The listing builds one solid part. Answer for the finished solid, in the listing's coordinates (mm). A direction names the side the tool comes from. Give positions to 0.01 mm unless a question says otherwise; leave off trailing zeros. Answer as a JSON object with one key per item and string values. Group by question number.
```python
from build123d import *

# Parameters (mm, degrees)
BOSS_EXTRUDE1_DEPTH = 102.5
FILLET1_R           = 1
CUT_EXTRUDE1_DEPTH  = 103.5
FILLET2_R           = 0.5
FILLET3_R           = 0.25


with BuildPart() as part:
    # Sketch3 → Boss-Extrude1 (new body)
    with BuildSketch(Plane(origin=(0, 0, 0), x_dir=(1, 0, 0), z_dir=(0, 1, 0))):
        with BuildLine():
            Line((7, 18.5), (7, 19.5))
            ThreePointArc((7, 19.5), (6.646446609, 19.646446609), (6.5, 20))
            Line((6.5, 20), (0, 20))
            Line((0, 20), (0, 13.5))
            ThreePointArc((0, 13.5), (0.353553391, 13.353553391), (0.5, 13))
            Line((0.5, 13), (1.5, 13))
            Line((1.5, 13), (1.5, 16))
            Line((1.5, 16), (3, 16))
            Line((3, 16), (5.5, 13.5))
            Line((5.5, 13.5), (5.5, 10.5))
            Line((5.5, 10.5), (6, 10))
            Line((6, 10), (5.5, 9.5))
            Line((5.5, 9.5), (5.5, 6.5))
            Line((5.5, 6.5), (3, 4))
            Line((3, 4), (1.5, 4))
            Line((1.5, 4), (1.5, 7))
            Line((1.5, 7), (0.5, 7))
            ThreePointArc((0.5, 7), (0.353553391, 6.646446609), (0, 6.5))
            Line((0, 6.5), (0, 0))
            Line((0, 0), (6.5, 0))
            ThreePointArc((6.5, 0), (6.646446609, 0.353553391), (7, 0.5))
            Line((7, 0.5), (7, 1.5))
            Line((7, 1.5), (4, 1.5))
            Line((4, 1.5), (4, 3))
            Line((4, 3), (6.5, 5.5))
            Line((6.5, 5.5), (9.5, 5.5))
            Line((9.5, 5.5), (10, 6))
            Line((10, 6), (10.5, 5.5))
            Line((10.5, 5.5), (13.5, 5.5))
            Line((13.5, 5.5), (16, 3))
            Line((16, 3), (16, 1.5))
            Line((16, 1.5), (13, 1.5))
            Line((13, 1.5), (13, 0.5))
            ThreePointArc((13, 0.5), (13.353553391, 0.353553391), (13.5, 0))
            Line((13.5, 0), (20, 0))
            Line((20, 0), (20, 6.5))
            ThreePointArc((20, 6.5), (19.646446609, 6.646446609), (19.5, 7))
            Line((19.5, 7), (18.5, 7))
            Line((18.5, 7), (18.5, 4))
            Line((18.5, 4), (17, 4))
            Line((17, 4), (14.5, 6.5))
            Line((14.5, 6.5), (14.5, 9.5))
            Line((14.5, 9.5), (14, 10))
            Line((14, 10), (14.5, 10.5))
            Line((14.5, 10.5), (14.5, 13.5))
            Line((14.5, 13.5), (17, 16))
            Line((17, 16), (18.5, 16))
            Line((18.5, 16), (18.5, 13))
            Line((18.5, 13), (19.5, 13))
            ThreePointArc((19.5, 13), (19.646446609, 13.353553391), (20, 13.5))
            Line((20, 13.5), (20, 20))
            Line((20, 20), (13.5, 20))
            ThreePointArc((13.5, 20), (13.353553391, 19.646446609), (13, 19.5))
            Line((13, 19.5), (13, 18.5))
            Line((13, 18.5), (16, 18.5))
            Line((16, 18.5), (16, 17))
            Line((16, 17), (13.5, 14.5))
            Line((13.5, 14.5), (10.5, 14.5))
            Line((10.5, 14.5), (10, 14))
            Line((10, 14), (9.5, 14.5))
            Line((9.5, 14.5), (6.5, 14.5))
            Line((6.5, 14.5), (4, 17))
            Line((4, 17), (4, 18.5))
            Line((4, 18.5), (7, 18.5))
        make_face()
    extrude(amount=BOSS_EXTRUDE1_DEPTH)

    # Fillet1
    fillet1_edges = [part.edges().sort_by_distance(p)[0] for p in [
        (20, 51.25, 0),
        (0, 51.25, 0),
        (0, 51.25, -20),
        (20, 51.25, -20),
    ]]
    fillet(fillet1_edges, radius=FILLET1_R)

    # Sketch4 → Cut-Extrude1 (cut, through all)
    with BuildSketch(Plane(origin=(0, 102.5, 0), x_dir=(1, 0, 0), z_dir=(0, 1, 0))):
        with BuildLine():
            Line((10, 11), (11.195582496, 12.195582496))
            ThreePointArc((11.195582496, 12.195582496), (10, 12.5), (8.804417504, 12.195582496))
            Line((8.804417504, 12.195582496), (10, 11))
        make_face()
        with BuildLine():
            ThreePointArc((12.195582496, 11.195582496), (11.767766953, 11.767766953), (11.195582496, 12.195582496))
            Line((11.195582496, 12.195582496), (10, 11))
            Line((10, 11), (11, 10))
            Line((11, 10), (12.195582496, 11.195582496))
        make_face()
        with BuildLine():
            Line((9, 10), (10, 11))
            Line((10, 11), (8.804417504, 12.195582496))
            ThreePointArc((8.804417504, 12.195582496), (8.232233047, 11.767766953), (7.804417504, 11.195582496))
            Line((7.804417504, 11.195582496), (9, 10))
        make_face()
        Polygon((11, 10), (10, 11), (9, 10), (10, 9), align=None)
        with BuildLine():
            Line((7.804417504, 8.804417504), (9, 10))
            Line((9, 10), (7.804417504, 11.195582496))
            ThreePointArc((7.804417504, 11.195582496), (7.5, 10), (7.804417504, 8.804417504))
        make_face()
        with BuildLine():
            Line((10, 9), (9, 10))
            Line((9, 10), (7.804417504, 8.804417504))
            ThreePointArc((7.804417504, 8.804417504), (8.232233047, 8.232233047), (8.804417504, 7.804417504))
            Line((8.804417504, 7.804417504), (10, 9))
        make_face()
        with BuildLine():
            Line((11.195582496, 7.804417504), (10, 9))
            Line((10, 9), (8.804417504, 7.804417504))
            ThreePointArc((8.804417504, 7.804417504), (10, 7.5), (11.195582496, 7.804417504))
        make_face()
        with BuildLine():
            Line((12.195582496, 8.804417504), (11, 10))
            Line((11, 10), (10, 9))
            Line((10, 9), (11.195582496, 7.804417504))
            ThreePointArc((11.195582496, 7.804417504), (11.767766953, 8.232233047), (12.195582496, 8.804417504))
        make_face()
        with BuildLine():
            ThreePointArc((12.5, 10), (12.422700584, 10.616864556), (12.195582496, 11.195582496))
            Line((12.195582496, 11.195582496), (11, 10))
            Line((11, 10), (12.195582496, 8.804417504))
            ThreePointArc((12.195582496, 8.804417504), (12.422700584, 9.383135444), (12.5, 10))
        make_face()
        with BuildLine():
            ThreePointArc((8.804417504, 7.804417504), (8.232233047, 8.232233047), (7.804417504, 8.804417504))
            Line((7.804417504, 8.804417504), (7, 8))
            Line((7, 8), (8, 7))
            Line((8, 7), (8.804417504, 7.804417504))
        make_face()
        with BuildLine():
            Line((13, 8), (12.195582496, 8.804417504))
            ThreePointArc((12.195582496, 8.804417504), (11.767766953, 8.232233047), (11.195582496, 7.804417504))
            Line((11.195582496, 7.804417504), (12, 7))
            Line((12, 7), (13, 8))
        make_face()
        with BuildLine():
            Line((13, 12), (12, 13))
            Line((12, 13), (11.195582496, 12.195582496))
            ThreePointArc((11.195582496, 12.195582496), (11.767766953, 11.767766953), (12.195582496, 11.195582496))
            Line((12.195582496, 11.195582496), (13, 12))
        make_face()
        with BuildLine():
            ThreePointArc((7.804417504, 11.195582496), (8.232233047, 11.767766953), (8.804417504, 12.195582496))
            Line((8.804417504, 12.195582496), (8, 13))
            Line((8, 13), (7, 12))
            Line((7, 12), (7.804417504, 11.195582496))
        make_face()
    extrude(amount=-CUT_EXTRUDE1_DEPTH, mode=Mode.SUBTRACT)

    # Fillet2
    fillet2_edges = [part.edges().sort_by_distance(p)[0] for p in [
        (18.5, 51.25, -13),
        (18.5, 51.25, -16),
        (14.5, 51.25, -10.5),
        (14.5, 51.25, -9.5),
        (18.5, 51.25, -4),
        (18.5, 51.25, -7),
        (13, 51.25, -1.5),
        (16, 51.25, -1.5),
        (10.5, 51.25, -5.5),
        (9.5, 51.25, -5.5),
        (4, 51.25, -1.5),
        (7, 51.25, -1.5),
        (1.5, 51.25, -7),
        (1.5, 51.25, -4),
        (5.5, 51.25, -9.5),
        (5.5, 51.25, -10.5),
        (1.5, 51.25, -16),
        (1.5, 51.25, -13),
        (7, 51.25, -18.5),
        (4, 51.25, -18.5),
        (9.5, 51.25, -14.5),
        (10.5, 51.25, -14.5),
        (16, 51.25, -18.5),
        (13, 51.25, -18.5),
    ]]
    fillet(fillet2_edges, radius=FILLET2_R)

    # Fillet3
    fillet3_edges = [part.edges().sort_by_distance(p)[0] for p in [
        (7, 51.25, -12),
        (8, 51.25, -13),
        (12, 51.25, -13),
        (13, 51.25, -12),
        (13, 51.25, -8),
        (12, 51.25, -7),
        (8, 51.25, -7),
        (7, 51.25, -8),
    ]]
    fillet(fillet3_edges, radius=FILLET3_R)


solid = part.part
```
Item 1: Determine the mould class of faces 1 (the flat face through (5, 51, -4)), 2 (the flat face through (0, 51, -4)), 3 (the flat face through (16, 51, 0)) for opening direction Z: released by +Z, released by -Z, zero draft, split by the parting line, or undercut.
Item 2: Consider probe 1 along Z at (x, y) = (15, 12.5); probe 2 along Z at (x, y) = (11.5, 12.5); probe 3 along X at (y, z) = (52, -8). Determine where each line is inside the solid, lowest interval first. Write a range as from..to.
Item 3: A tool of negligible diameter and unlimited length cuts with its end or side. For faces 4 (the flat face through (4, 51, -20)), 5 (the flat face through (15, 51, -4)), from which of +Z, -Z, +X, -X, +Y, -Y can it reach the whole face along a straight path? Write none if from no direction.
Item 4: Flat-ended cylindrical pins translate along their axes: P1, Ø1.4, axis at x = 11.5, y = 50.5, coming from the +Z side; P2, Ø3, axis at y = 58.5, z = -12.5, coming from the -X side; P3, Ø1.4, axis at y = 38.5, z = -8.5, coming from the +X side. Find the tip coordinate at first contact, or state that the pin passes through.
Values found:
{
 "1": {"face 1": "undercut", "face 2": "zero draft", "face 3": "released by +Z"},
 "2": {"probe 1": "z = -20..-18.5, -16..-14, -6..-4, -1.5..0", "probe 2": "z = -14.5..-12.5, -7.5..-5.5", "probe 3": "x = 5.5..7.1, 12.9..14.5"},
 "3": {"face 4": "-Z, +X, -X, +Y, -Y", "face 5": "+Y, -Y"},
 "4": {"P1": "stops at z = -5.5", "P2": "stops at x = 0", "P3": "stops at x = 14.5"}
}
